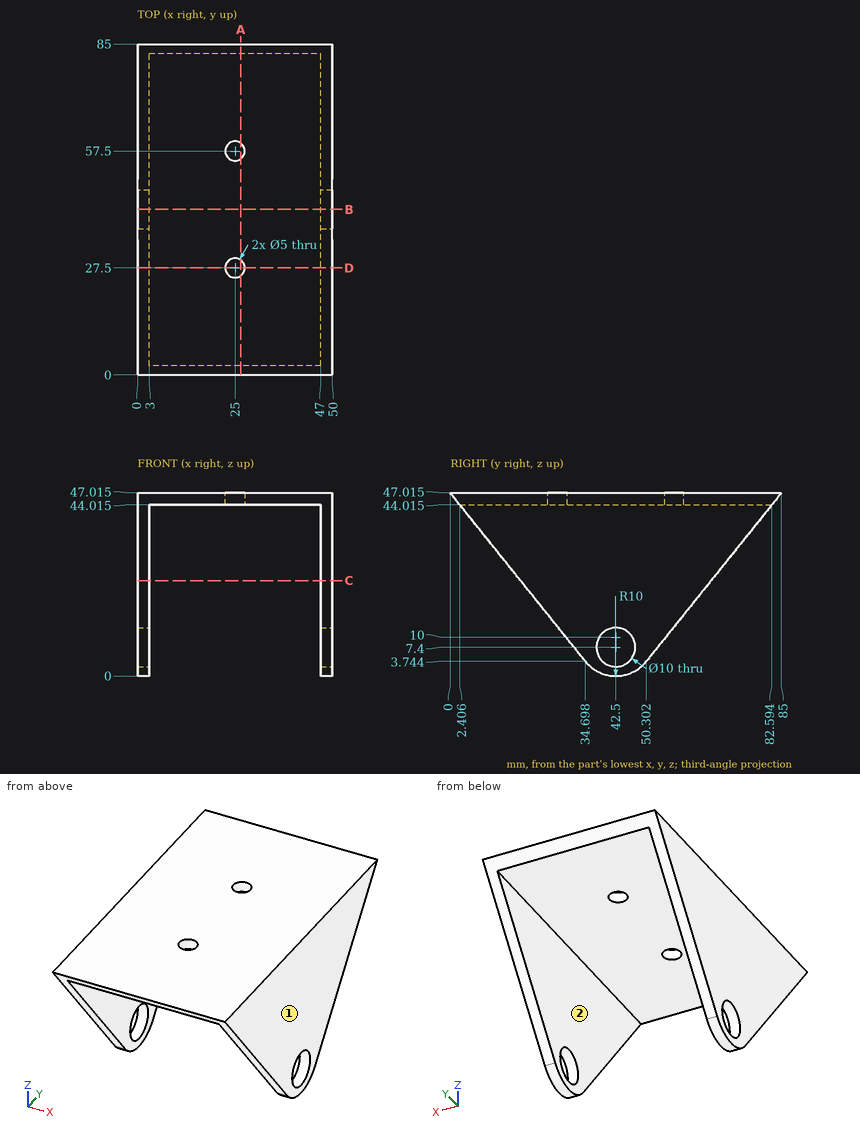
Design review of the part shown in the three views and the two pictorial views. Dimensions are in mm from the part's minimum x, y and z. A direction names the side the tool comes from. Round coordinates to 2 decimals unless told otherwise and drop trailing zeros. Loops run counter-clockwise (first coordinate to the right, second up) from the corner with the lowest first, then second, coordinate; pieces in that order, holes last. Notation, with made-up numbers: M 39,-7 L 47,-7 A10 cw 47,-3 Z; hole C 12,56.25 d5. An arc over 180 degrees is marked long. Answer as a JSON object with one key per item and string values.
Item 1: We need section A-A on x = 26.5. Give the boundary of the cut face in (y, z) (1 decimal), and give its area (3 significant figures).
Answer sheet:
{"outline": "M 0,47 L 2.4,44 L 25.5,44 L 25.5,47 Z; M 29.5,44 L 55.5,44 L 55.5,47 L 29.5,47 Z; M 59.5,44 L 82.6,44 L 85,47 L 59.5,47 Z", "area": "224 mm^2"}
Item 2: Machinability: for the marked faces 1 and 2, which of the approach directions +Z, -Z, +X, -X, +Y, -Y give a long, thin tool a straight path to every point of the face, cutting with its end or side? Answer none if there is none.
Answer sheet:
{"face 1": "+Z, -Z, +X, +Y, -Y", "face 2": "-Z, +Y, -Y"}
Item 3: We need section D-D on y = 27.5. Give the boundary of the cut face in (x, z) (1 decimal).
Answer sheet:
{"outline": "M 0,12.7 L 3,12.7 L 3,44 L 22.5,44 L 22.5,47 L 0,47 Z; M 27.5,44 L 47,44 L 47,12.7 L 50,12.7 L 50,47 L 27.5,47 Z"}
Item 4: Clearance check with flat-ended pins moving along their axes: P1, Ø3, axis at y = 17.5, z = 22, coming from the +X side; P2, Ø8, axis at x = 25, y = 48.5, coming from the -Z side (1 decimal). State where each tip first meets the part, or that it passes through.
Answer sheet:
{"P1": "passes through", "P2": "stops at z = 44"}
Item 5: We need section B-B on y = 42.5. Give the boundary of the cut face in (x, z) (1 decimal).
Answer sheet:
{"outline": "M 0,0 L 3,0 L 3,2.4 L 0,2.4 Z; M 0,12.4 L 3,12.4 L 3,44 L 47,44 L 47,12.4 L 50,12.4 L 50,47 L 0,47 Z; M 47,0 L 50,0 L 50,2.4 L 47,2.4 Z"}
Item 6: Wall thickness on L1, parallel to X at y = 58.5, z = 38; L2, parallel to Y at x = 25, z = 45 (1 decimal); L3, parallel to Z at x = 17.5, y = 44.5 (1 decimal): over which ranges is each line inside the solid? List them lowest first. Write a range as from..to.
Answer sheet:
{"L1": "x = 0..3, 47..50", "L2": "y = 1.6..25, 30..55, 60..83.4", "L3": "z = 44..47"}
Item 7: We need section C-C on z = 24.5. Give the boundary of the cut face in (x, y) (1 decimal).
Answer sheet:
{"outline": "M 0,18.1 L 3,18.1 L 3,66.9 L 0,66.9 Z; M 47,18.1 L 50,18.1 L 50,66.9 L 47,66.9 Z"}
